```python
from build123d import *

# Parameters (mm, degrees)
SKETCH1_R           = 6
BOSS_EXTRUDE1_DEPTH = 10
FILLET1_R           = 0.5
SKETCH2_OUTSIDE_W   = 17.94
SKETCH2_OUTSIDE_H   = 17.94
SKETCH2_OUTSIDE_R   = 5.5
CUT_EXTRUDE11_DEPTH = 0.5
SKETCH3_R           = 5
CUT_EXTRUDE12_DEPTH = 4


with BuildPart() as part:
    # Sketch1 → Boss-Extrude1 (new body)
    with BuildSketch(Plane(origin=(0, 0, 0), x_dir=(1, 0, 0), z_dir=(0, 1, 0))):
        Circle(SKETCH1_R)
    extrude(amount=BOSS_EXTRUDE1_DEPTH)

    # Fillet1
    fillet1_edges = [part.edges().sort_by_distance(p)[0] for p in [
        (-6, 10, 0),
    ]]
    fillet(fillet1_edges, radius=FILLET1_R)

    # Sketch2 outside → Cut-Extrude11 (cut)
    with BuildSketch(Plane(origin=(0, 0, 0), x_dir=(1, 0, 0), z_dir=(0, 1, 0))):
        Rectangle(SKETCH2_OUTSIDE_W, SKETCH2_OUTSIDE_H)
        Circle(SKETCH2_OUTSIDE_R, mode=Mode.SUBTRACT)
    extrude(amount=CUT_EXTRUDE11_DEPTH, mode=Mode.SUBTRACT)

    # Sketch3 → Cut-Extrude12 (cut)
    with BuildSketch(Plane(origin=(0, 10, 0), x_dir=(1, 0, 0), z_dir=(0, 1, 0))):
        Circle(SKETCH3_R)
    extrude(amount=-CUT_EXTRUDE12_DEPTH, mode=Mode.SUBTRACT)


solid = part.part
```
Here's how the part is built. I have some questions about the finished solid (model axes, mm). A direction names the side the tool comes from. Round coordinates to 2 decimals unless told otherwise and drop trailing zeros. Order: outer loops, then holes, each group sorted by start corner. A loop starts at its lowest first (then second) coordinate and runs counter-clockwise, first axis right, second up. Notation, with made-up numbers: (20.5, 87.25) -> (44.5, 87.25) arc R14 cw to (44.5, 103.25) -> close; hole circle Ø7 at (82.5, -23). An arc over 180 degrees is marked (long way). Use a Markdown table: item, result. Add a question column.
(1) If we mould it in two halves opening along X, with no side actions, what happens to faces 1 (the face through (-1.19, 0.25, 5.37)), 2 (the face through (0, 6, 0)), 3 (the face through (1.6, 10, 4.9)), 4 (the face through (-1.08, 8.03, 4.88))? For each: released by +X, released by -X, zero draft, split by the parting line, or undercut.
(2) Suppose I cut it at B-B, the plane z = 0. Please give me the cut outline in (x, y).
(3) I need wall thicknesses on line 1 along X through (y, z) = (8.35, 0); line 2 along Y through (x, z) = (1, -4.75). Which ranges of each line are inside material? Lowest first, please.
(4) For pin 1 Ø1.5 at (y, z) = (3.5, -1) entering from +X; pin 2 Ø1 at (x, z) = (-3.5, -4.5) entering from +Y; pin 3 Ø3 at (y, z) = (3, 5) entering from +X, each with a flat end and sliding along its axis, tell me the tip position at first contact or that it passes through.
(5) Suppose I cut it at A-A, the plane x = 0. Please give me the cut outline in (y, z), and give its area (3 significant figures).
(6) Suppose I cut it at D-D, the plane y = 4. Please give me the cut outline in (x, z), and give its area (3 significant figures).
(7) Suppose I cut it at C-C, the plane y = 8.5. Please give me the cut outline in (x, z).
(8) For faces 5 (the face through (0, 0, 0)), 6 (the face through (3, 0.5, 5)), which set-ups out of +Z, -Z, +X, -X, +Y, -Y let a thin tool reach every point of the face, with its end or its side?
Verdict:
| question | item | result |
|---|---|---|
| 1 | face 1 | split by the parting line |
| 1 | face 2 | undercut |
| 1 | face 3 | zero draft |
| 1 | face 4 | undercut |
| 2 | outline | (-6, 0.5) -> (-5.5, 0.5) -> (-5.5, 0) -> (5.5, 0) -> (5.5, 0.5) -> (6, 0.5) -> (6, 9.5) arc R0.5 ccw to (5.5, 10) -> (5, 10) -> (5, 6) -> (-5, 6) -> (-5, 10) -> (-5.5, 10) arc R0.5 ccw to (-6, 9.5) -> close |
| 3 | line 1 | -6 to -5, 5 to 6 |
| 3 | line 2 | 0 to 6 |
| 4 | pin 1 | x = 5.99 |
| 4 | pin 2 | y = 10 |
| 4 | pin 3 | x = 4.87 |
| 5 | outline | (0, -5.5) -> (0.5, -5.5) -> (0.5, -6) -> (9.5, -6) arc R0.5 ccw to (10, -5.5) -> (10, -5) -> (6, -5) -> (6, 5) -> (10, 5) -> (10, 5.5) arc R0.5 ccw to (9.5, 6) -> (0.5, 6) -> (0.5, 5.5) -> (0, 5.5) -> close |
| 5 | area | 79.4 mm2 |
| 6 | outline | circle Ø12 at (0, 0) |
| 6 | area | 113 mm2 |
| 7 | outline | circle Ø12 at (0, 0); hole circle Ø10 at (0, 0) |
| 8 | face 5 | +Z, -Z, +X, -X, -Y |
| 8 | face 6 | -Y |
